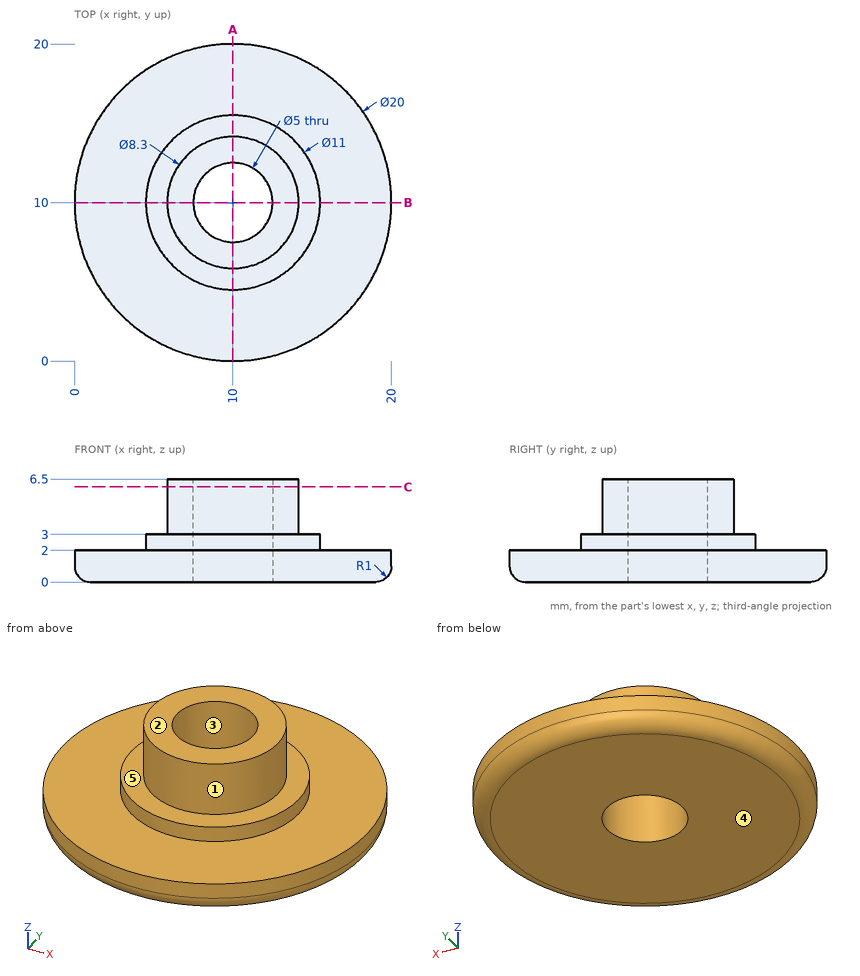
Geometry check sheet. Reference: drawing and pictorial views, mm from the part's lowest x, y, z. A direction names the side the tool comes from. Coordinates: 2 decimals unless noted, no trailing zeros. Loops run counter-clockwise (first coordinate to the right, second up) from the corner with the lowest first, then second, coordinate; pieces in that order, holes last. Notation, with made-up numbers: M 43.25,17 L 79.25,17 A33 cw 79.25,49 Z; hole C 1,-7 d1. An arc over 180 degrees is marked long. One line per item, written item: value.
1. Mould release check, pull along X, two halves, no side actions. Record for the marked faces 1, 2 and 3: pulls with the +X half, pulls with the -X half, needs draft (parallel to the pull), parting line crosses it, or undercut.
Answers follow:
face 1: parting line crosses it
face 2: needs draft
face 3: undercut
2. Gauge pin test, flat ends, axial feed: P1, Ø3, axis at y = 5, z = 1.5, coming from the -X side; P2, Ø3, axis at x = 13.5, y = 3.5, coming from the +Z side; P3, Ø3, axis at y = 3.5, z = 1, coming from the -X side. Record the tip position at first contact, or that the pin passes through.
Answers follow:
P1: x = 0.63
P2: z = 2
P3: x = 1.34
3. Section check C-C on z = 6. Record the cut outline in (x, y), plus the area to 3 significant figures.
Answers follow:
outline: C 10,10 d8.3; hole C 10,10 d5
area: 34.5 mm^2
4. Section check A-A on x = 10. Record the cut outline in (y, z), plus the area to 3 significant figures.
Answers follow:
outline: M 0,1 A1 ccw 1,0 L 7.5,0 L 7.5,6.5 L 5.85,6.5 L 5.85,3 L 4.5,3 L 4.5,2 L 0,2 Z; M 12.5,0 L 19,0 A1 ccw 20,1 L 20,2 L 15.5,2 L 15.5,3 L 14.15,3 L 14.15,6.5 L 12.5,6.5 Z
area: 47.1 mm^2
5. Set-up check for the marked faces 4 and 5: record each of +Z, -Z, +X, -X, +Y, -Y from which the full face is reachable in a straight line by a thin tool's end or side.
Answers follow:
face 4: -Z, +X, -X, +Y, -Y
face 5: +Z
6. Material ranges on line 1 along Y through (x, z) = (10, 4.5); line 2 along Y through (x, z) = (10, 1.5); line 3 along Z through (x, y) = (16.5, 13), recorded low to high. Write a range as from..to.
Answers follow:
line 1: 5.85..7.5, 12.5..14.15
line 2: 0..7.5, 12.5..20
line 3: 0..2
